```python
from build123d import *

# Parameters (mm, degrees)
SKETCH1_W           = 33.537053001
SKETCH1_H           = 60
BOSS_EXTRUDE1_DEPTH = 10
SKETCH2_R           = 1.35
CUT_EXTRUDE1_DEPTH  = 10
CUT_EXTRUDE3_DEPTH  = 18
SKETCH10_W          = 20.892081227
SKETCH10_H          = 64.192604416
CUT_EXTRUDE4_DEPTH  = 26
SKETCH15_W          = 6.200817496
SKETCH15_H          = 60
CUT_EXTRUDE5_DEPTH  = 26
FILLET1_R           = 1
SKETCH16_R          = 2.5
CUT_EXTRUDE6_DEPTH  = 2


with BuildPart() as part:
    # Sketch1 → Boss-Extrude1 (new body)
    with BuildSketch(Plane(origin=(0, 0, 0), x_dir=(1, 0, 0), z_dir=(0, 1, 0))):
        with Locations((16.768526501, 0)):
            Rectangle(SKETCH1_W, SKETCH1_H)
    extrude(amount=BOSS_EXTRUDE1_DEPTH)

    # Sketch2 → Cut-Extrude1 (cut)
    with BuildSketch(Plane.ZY):
        with Locations((-6.75, 5)):
            Circle(SKETCH2_R)
        with Locations(Location((6.75, 5, 0), (0, 0, 180))):
            Circle(SKETCH2_R)
    extrude(amount=-CUT_EXTRUDE1_DEPTH, mode=Mode.SUBTRACT)

    # Sketch5 → Cut-Extrude3 (cut)
    with BuildSketch(Plane(origin=(0, 10, 0), x_dir=(1, 0, 0), z_dir=(0, 1, 0))):
        Polygon((0, 13.591085099), (4.530530491, 30), (0, 30), align=None)
        Polygon((0, -30), (4.530530491, -30), (0, -13.591085099), align=None)
    extrude(amount=-CUT_EXTRUDE3_DEPTH, mode=Mode.SUBTRACT)

    # Sketch10 → Cut-Extrude4 (cut)
    with BuildSketch(Plane(origin=(0, 10, 0), x_dir=(1, 0, 0), z_dir=(0, 1, 0))):
        with Locations((23.64685811, -0.926664893)):
            Rectangle(SKETCH10_W, SKETCH10_H)
    extrude(amount=-CUT_EXTRUDE4_DEPTH, mode=Mode.SUBTRACT)

    # Sketch15 → Cut-Extrude5 (cut)
    with BuildSketch(Plane(origin=(0, 10, 0), x_dir=(1, 0, 0), z_dir=(0, 1, 0))):
        with Locations((10.100408748, 0)):
            Rectangle(SKETCH15_W, SKETCH15_H)
    extrude(amount=-CUT_EXTRUDE5_DEPTH, mode=Mode.SUBTRACT)

    # Fillet1
    fillet1_edges = [part.edges().sort_by_distance(p)[0] for p in [
        (5.765265246, 0, -30),
        (5.765265246, 10, -30),
        (4.530530491, 5, -30),
        (4.530530491, 5, 30),
        (7, 5, 30),
        (7, 5, -30),
    ]]
    fillet(fillet1_edges, radius=FILLET1_R)

    # Sketch16 → Cut-Extrude6 (cut)
    with BuildSketch(Plane(origin=(7, 0, 0), x_dir=(0, 0, -1), z_dir=(1, 0, 0))):
        with Locations((-6.75, 5)):
            Circle(SKETCH16_R)
        with Locations((6.75, 5)):
            Circle(SKETCH16_R)
    extrude(amount=-CUT_EXTRUDE6_DEPTH, mode=Mode.SUBTRACT)


solid = part.part
```
Part model, mm, in its own coordinate system. A direction names the side the tool comes from. Coordinates: 2 decimals unless noted, no trailing zeros. Order: outer loops, then holes, each group sorted by start corner. A loop starts at its lowest first (then second) coordinate and runs counter-clockwise, first axis right, second up. Notation, with made-up numbers: (41.5, 10.25) - (95.5, 10.25) arc R9 cw to (95.5, 14.25) - close; hole circle Ø2 at (-38.75, 82). An arc over 180 degrees is marked (long way). Return JSON: item names as keys, results as strings. Group by question number.
Item 1: Pull direction Z, two halves, no side cores. Call faces 3 (the face through (2.465, 5.406, -5.462)), 4 (the face through (6.715, 4.93, 29.699)), 5 (the face through (2.134, 5.07, -21.319)): pulls with the +Z half, pulls with the -Z half, needs draft (parallel to the pull), parting line crosses it, or undercut.
Item 2: Pin check, flat tips, straight feed: pin 1 (1.5 mm diameter, centred on y = 5.5, z = 17.5, fed in from -X); pin 2 (4 mm diameter, centred on x = 2.5, y = 6.5, fed in from -Z); pin 3 (2.5 mm diameter, centred on y = 5, z = -7, fed in from +X). Stop position of each tip, or through.
Item 3: Cut at D-D (x = 1.25). List the corners of the cut face in (y, z).
Item 4: Drill centre lines: probe 1 along Y at (x, z) = (2.5, -6.75); probe 2 along Y at (x, z) = (5.65, 6.75); probe 3 along X at (y, z) = (7.25, 6). Where is each one in solid material? Low to high. Write a range as from..to.
Item 5: Which spindle directions (+Z, -Z, +X, -X, +Y, -Y) get a long thin tool onto all of the face, cutting with end or side? Do faces 1 (the face through (5.6, 0.2, -29.6)), 2 (the face through (6.014, 5.751, -9.135)). Say none if no direction does.
Item 6: Cut at C-C (y = 1.5). List the corners of the cut face in (x, z), plus the area to 3 significant figures.
Item 7: Cut at B-B (z = 6.75). List the corners of the cut face in (x, y), plus the area to 3 significant figures.
Item 8: Cut at A-A (y = 5). List the corners of the cut face in (x, z), plus the area to 3 significant figures.
Check values:
{
 "1": {"face 3": "undercut", "face 4": "pulls with the +Z half", "face 5": "pulls with the -Z half"},
 "2": {"pin 1": "stops at x = 0.87", "pin 2": "stops at z = -29.61", "pin 3": "stops at x = 5"},
 "3": {"outline": "(0, -18.12) - (10, -18.12) - (10, 18.12) - (0, 18.12) - close; hole circle Ø2.7 at (5, -6.75); hole circle Ø2.7 at (5, 6.75)"},
 "4": {"probe 1": "y = 0..3.65, 6.35..10", "probe 2": "y = 0..2.5, 7.5..10", "probe 3": "x = 0..5"},
 "5": {"face 1": "-Z, +X, -X, -Y", "face 2": "+X"},
 "6": {"outline": "(0, -13.59) - (4.33, -29.27) arc R1 ccw to (5.29, -30) - (6, -30) arc R1 ccw to (7, -29) - (7, 29) arc R1 ccw to (6, 30) - (5.29, 30) arc R1 ccw to (4.33, 29.27) - (0, 13.59) - close", "area": "345 mm2"},
 "7": {"outline": "(0, 0) - (7, 0) - (7, 2.5) - (5, 2.5) - (5, 3.65) - (0, 3.65) - close; (0, 6.35) - (5, 6.35) - (5, 7.5) - (7, 7.5) - (7, 10) - (0, 10) - close", "area": "46.5 mm2"},
 "8": {"outline": "(0, -13.59) - (4.33, -29.27) arc R1 ccw to (5.29, -30) - (6, -30) arc R1 ccw to (7, -29) - (7, -9.25) - (5, -9.25) - (5, -8.1) - (0, -8.1) - close; (0, -5.4) - (5, -5.4) - (5, -4.25) - (7, -4.25) - (7, 4.25) - (5, 4.25) - (5, 5.4) - (0, 5.4) - close; (0, 8.1) - (5, 8.1) - (5, 9.25) - (7, 9.25) - (7, 29) arc R1 ccw to (6, 30) - (5.29, 30) arc R1 ccw to (4.33, 29.27) - (0, 13.59) - close", "area": "298 mm2"}
}
